from build123d import *

# Parameters (mm, degrees)
SKETCH_1_W      = 130
SKETCH_1_H      = 130
SKETCH_1_R      = 1.25
EXTRUDE_1_DEPTH = 2


with BuildPart() as part:
    # Эскиз1 → Бобышка-Вытянуть1 (new body)
    with BuildSketch(Plane.XY):
        Rectangle(SKETCH_1_W, SKETCH_1_H)
        with Locations((-55, 55)):
            Circle(SKETCH_1_R, mode=Mode.SUBTRACT)
        with Locations((55, 50)):
            Circle(SKETCH_1_R, mode=Mode.SUBTRACT)
        with Locations((55, -55)):
            Circle(SKETCH_1_R, mode=Mode.SUBTRACT)
        with Locations((-55, -50)):
            Circle(SKETCH_1_R, mode=Mode.SUBTRACT)
        with BuildLine():
            Line((-18.999998719, 10.000001538), (-18.999998719, -9.000007164))
            Line((-18.999998719, -9.000007164), (19.000000929, -9.000007164))
            Line((19.000000929, -9.000007164), (19.000000929, 10.000001538))
            ThreePointArc((19.000000929, 10.000001538), (1.105e-06, 29.000001361), (-18.999998719, 10.000001538))
        make_face(mode=Mode.SUBTRACT)
    extrude(amount=EXTRUDE_1_DEPTH)


solid = part.part
The listing builds one solid part. Answer for the finished solid, in the listing's coordinates (mm). Coordinates: 2 decimals unless noted, no trailing zeros. Order: outer loops, then holes, each group sorted by start corner. A loop starts at its lowest first (then second) coordinate and runs counter-clockwise, first axis right, second up. Notation, with made-up numbers: M -31,-2 L -20,-2 A28 cw -20,17 Z; hole C 83,-18.5 d4. An arc over 180 degrees is marked long. Use CSV: the item, a comma, the result in double quotes.
Q1. Given pin 1 Ø2 at (x, y) = (-55, -50) entering from -Z, flat-ended and moving along its own axis, determine where the tip first touches the part or whether it passes through.
Here are the results:
pin 1,"through"
Q2. Straight lines are drawn through the part: L1, parallel to Y at x = 55, z = 1.4; L2, parallel to Y at x = -55, z = 1; L3, parallel to X at y = -7.5, z = 1. For each, find the intervals that lie inside material, in ascending order.
Here are the results:
L1,"-65 to -56.25, -53.75 to 48.75, 51.25 to 65"
L2,"-65 to -51.25, -48.75 to 53.75, 56.25 to 65"
L3,"-65 to -19, 19 to 65"
Q3. Section B-B (x = -5) is taken. Determine the outline of the cut face in (y, z).
Here are the results:
outline,"M -65,0 L -9,0 L -9,2 L -65,2 Z; M 28.33,0 L 65,0 L 65,2 L 28.33,2 Z"
Q4. Section C-C (y = 4.5) is taken. Determine the outline of the cut face in (x, z).
Here are the results:
outline,"M -65,0 L -19,0 L -19,2 L -65,2 Z; M 19,0 L 65,0 L 65,2 L 19,2 Z"
Q5. Section A-A (z = 1.4) is taken. Determine the outline of the cut face in (x, y), then the cut area to 3 significant figures.
Here are the results:
outline,"M -65,-65 L 65,-65 L 65,65 L -65,65 Z; hole C -55,-50 d2.5; hole C -55,55 d2.5; hole M -19,-9 L 19,-9 L 19,10 A19 ccw -19,10 Z; hole C 55,-55 d2.5; hole C 55,50 d2.5"
area,"15,600 mm2"
Q6. Determine the mould class of faces 1 (the flat face through (-1, -14, 2)), 2 (the cylindrical face through (0, 29, 1)) for opening direction Y: pulls with the +Y half, pulls with the -Y half, needs draft (parallel to the pull), parting line crosses it, or undercut.
Here are the results:
face 1,"needs draft"
face 2,"undercut"
